Geometry: see drawing. Coordinates: mm, zero at the bounding-box minimum. Give positions to 0.01 mm unless a question says otherwise; leave off trailing zeros. Loops run counter-clockwise (first coordinate to the right, second up) from the corner with the lowest first, then second, coordinate; pieces in that order, holes last. Notation, with made-up numbers: M 9,70 L 48,70 A22 ccw 48,102 Z; hole C 3.5,25.5 d7. An arc over 180 degrees is marked long. Put each result on its own line as item: value.
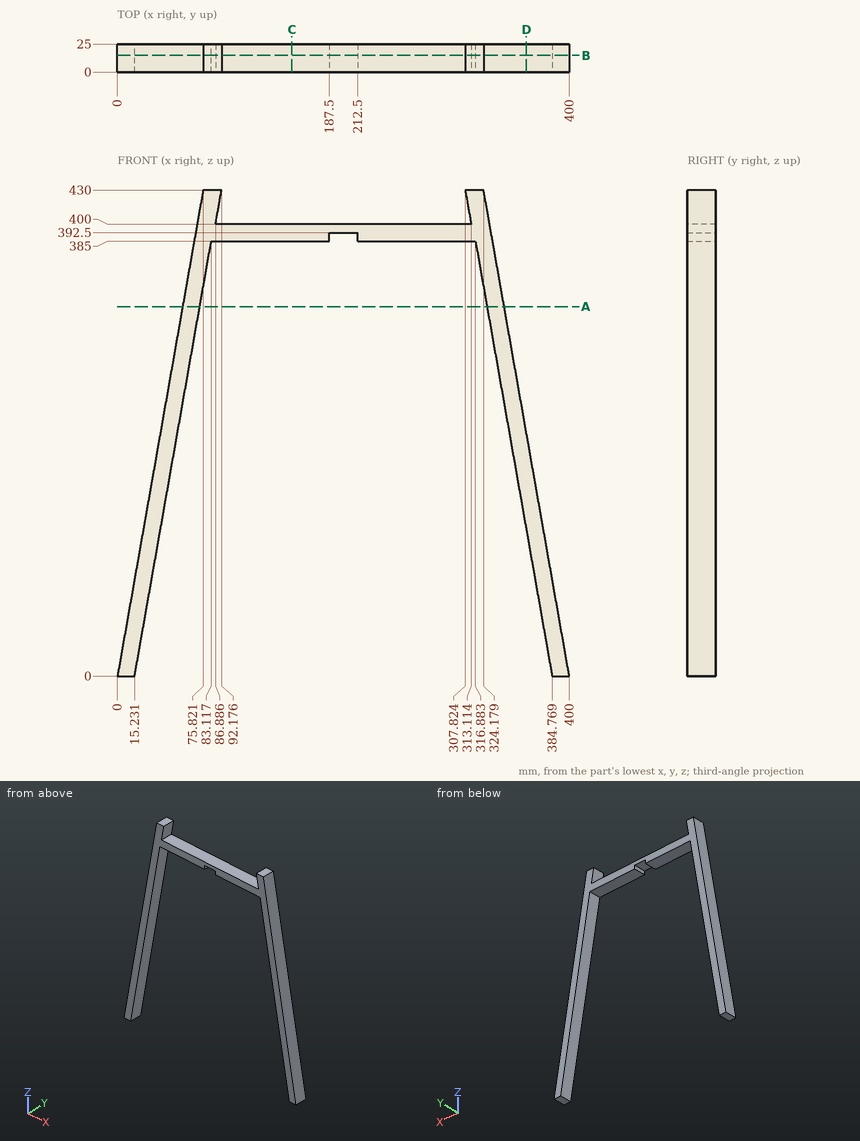
Item 1: Section A-A on z = 327. Output: boundary loops of the cut face in (x, y).
Output values:
outline: M 57.66,0 L 72.89,0 L 72.89,25 L 57.66,25 Z; M 327.11,0 L 342.34,0 L 342.34,25 L 327.11,25 Z
Item 2: Section C-C on x = 154.5. Output: boundary loops of the cut face in (y, z).
Output values:
outline: M 0,385 L 25,385 L 25,400 L 0,400 Z
Item 3: Line query: probe 1 along Z at (x, y) = (204.5, 8.75); probe 2 along Z at (x, y) = (284, 13); probe 3 along X at (y, z) = (22, 369) (1 decimal). Output: solid intervals per line, ascending. Write a range as [from, to].
Output values:
probe 1: [392.5, 400]
probe 2: [385, 400]
probe 3: [65.1, 80.3], [319.7, 334.9]
Item 4: Section B-B on y = 15. Output: boundary loops of the cut face in (x, z), then the cut area to 3 significant figures.
Output values:
outline: M 0,0 L 15.23,0 L 83.12,385 L 187.5,385 L 187.5,392.5 L 212.5,392.5 L 212.5,385 L 316.88,385 L 384.77,0 L 400,0 L 324.18,430 L 307.82,430 L 313.11,400 L 86.89,400 L 92.18,430 L 75.82,430 Z
area: 16,400 mm²
Item 5: Pin query (flat end, axial travel): pin 1 Ø3 at (y, z) = (18.5, 157.5) entering from -X; pin 2 Ø2 at (x, y) = (256.5, 6.5) entering from -Z; pin 3 Ø8 at (y, z) = (17.5, 131) entering from +X. Return the tip coordinate at first contact, or that it passes through.
Output values:
pin 1: x = 27.51
pin 2: z = 385
pin 3: x = 377.61
Item 6: Section D-D on x = 362. Output: boundary loops of the cut face in (y, z).
Output values:
outline: M 0,129.13 L 25,129.13 L 25,215.51 L 0,215.51 Z
